Study the drawing (mm; zero at the part's minimum x, y, z) and answer. Coordinates: 2 decimals unless noted, no trailing zeros. Loops run counter-clockwise (first coordinate to the right, second up) from the corner with the lowest first, then second, coordinate; pieces in that order, holes last. Notation, with made-up numbers: (49.25, 20) - (105.25, 20) arc R24 cw to (105.25, 43) - close; hole circle Ø7 at (-16.75, -21). An arc over 180 degrees is marked (long way). Put each result on its own line as item: value.
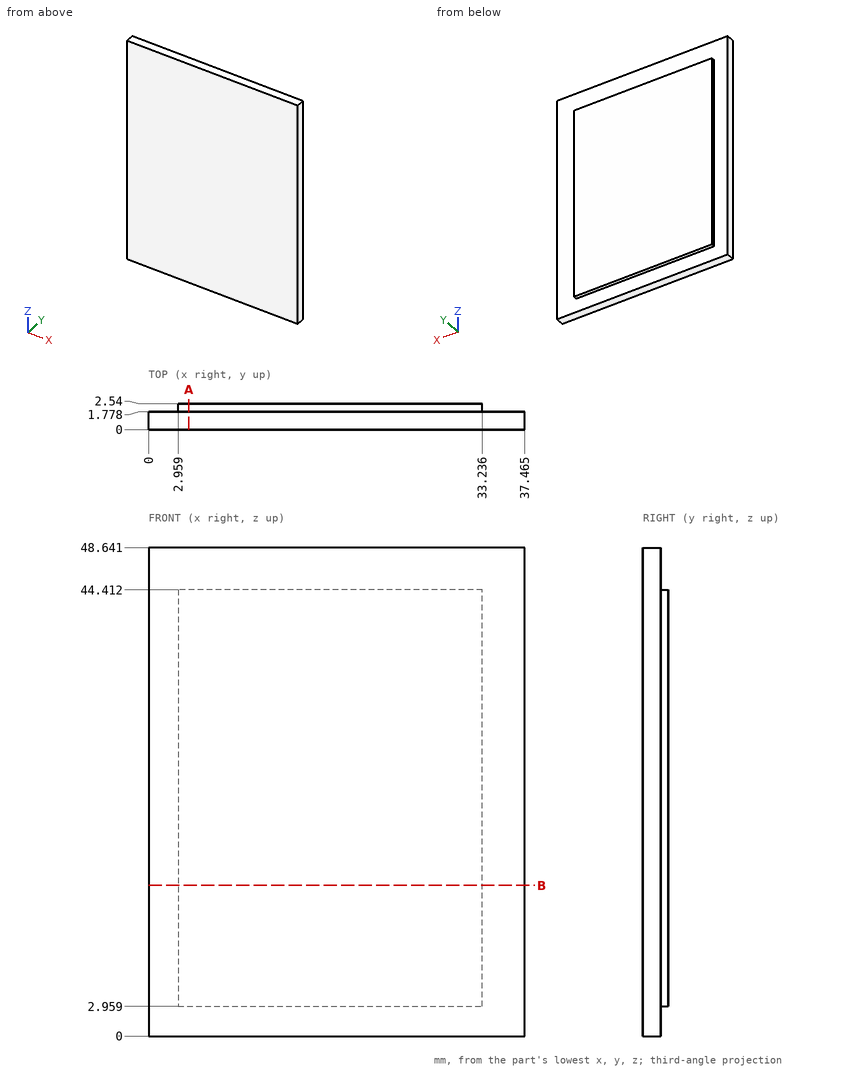
1) The part is cut by section B-B (z = 15). Give the vertices of the cut face in (x, y) (3 decimals), and give its area (3 significant figures).
Found:
outline: (0, 0) - (37.465, 0) - (37.465, 1.778) - (33.236, 1.778) - (33.236, 2.54) - (2.959, 2.54) - (2.959, 1.778) - (0, 1.778) - close
area: 89.7 mm^2
2) Straight lines are drawn through the part: L1, parallel to Y at x = 35, z = 30; L2, parallel to X at y = 1.85, z = 15; L3, parallel to Z at x = 12, y = 2.35. For each, find the intervals that lie inside material, in ascending order. Write a range as [from, to].
Found:
L1: y = [0, 1.78]
L2: x = [2.96, 33.24]
L3: z = [2.96, 44.41]
3) The part is cut by section A-A (x = 4). Give the vertices of the cut face in (y, z).
Found:
outline: (0, 0) - (1.78, 0) - (1.78, 2.96) - (2.54, 2.96) - (2.54, 44.41) - (1.78, 44.41) - (1.78, 48.64) - (0, 48.64) - close
